Read the model definition and answer for the solid it produces. Units are mm, in the model's axes. A direction names the side the tool comes from. Give positions to 0.01 mm unless a question says otherwise; leave off trailing zeros. Write each loop counter-clockwise with the first axis right and the second up, starting at its lowest first coordinate (ties: lowest second). Pieces come first, ordered by that corner, then holes.
```python
from build123d import *

# Parameters (mm, degrees)
EXTRUDE_1_DEPTH               = 5
HOLE_WIZARD_M10_1_D           = 11
HOLE_WIZARD_M10_1_CBORE_D     = 12.05
HOLE_WIZARD_M10_1_CBORE_DEPTH = 4
HOLE_WIZARD_M10_2_D           = 11
HOLE_WIZARD_M10_2_CBORE_D     = 12.05
HOLE_WIZARD_M10_2_CBORE_DEPTH = 4
FILLET_1_R                    = 2


with BuildPart() as part:
    # 草图1 → 凸台-拉伸1 (new body)
    with BuildSketch(Plane(origin=(0, 0, 0), x_dir=(-1, 0, 0), z_dir=(0, 0, -1))):
        with BuildLine():
            Line((-3, 22.583801513), (-3, 7.416198487))
            ThreePointArc((-3, 7.416198487), (0, -8), (3, 7.416198487))
            Line((3, 7.416198487), (3, 22.583801513))
            ThreePointArc((3, 22.583801513), (0, 38), (-3, 22.583801513))
        make_face()
    extrude(amount=-EXTRUDE_1_DEPTH)

    # M10 六角头螺栓的柱形沉头孔1 (through all)
    with Locations(Plane(origin=(0, 0, 0), x_dir=(-1, 0, 0), z_dir=(0, 0, -1))):
        with Locations((0, 30)):
            CounterBoreHole(HOLE_WIZARD_M10_1_D / 2, HOLE_WIZARD_M10_1_CBORE_D / 2, HOLE_WIZARD_M10_1_CBORE_DEPTH)

    # M10 六角头螺栓的柱形沉头孔2 (through all)
    with Locations(Plane.XY.offset(5)):
        with Locations((0, 0)):
            CounterBoreHole(HOLE_WIZARD_M10_2_D / 2, HOLE_WIZARD_M10_2_CBORE_D / 2, HOLE_WIZARD_M10_2_CBORE_DEPTH)

    # 圆角1
    fillet_1_edges = [part.edges().sort_by_distance(p)[0] for p in [
        (-3, 22.583801513, 2.5),
        (-3, 7.416198487, 2.5),
        (3, 7.416198487, 2.5),
        (3, 22.583801513, 2.5),
    ]]
    fillet(fillet_1_edges, radius=FILLET_1_R)


solid = part.part
```
Item 1: Section D-D (y = 1.5) is taken. Write down the section's boundary in (x, z).
Result set:
outline: (-7.86, 0) - (-5.29, 0) - (-5.29, 1) - (-5.84, 1) - (-5.84, 5) - (-7.86, 5) - close; (5.29, 0) - (7.86, 0) - (7.86, 5) - (5.84, 5) - (5.84, 1) - (5.29, 1) - close
Item 2: Each of these flat-tipped pins is pushed along its axis until it touches: pin 1 Ø9.5 at (x, y) = (0, 0) entering from +Z; pin 2 Ø1 at (x, z) = (-3.5, 4.5) entering from -Y; pin 3 Ø1.5 at (y, z) = (23.5, 3) entering from -X. Where does it stop, or does it pass through?
Result set:
pin 1: passes through
pin 2: stops at y = -7.42
pin 3: stops at x = -5.56
Item 3: Section C-C (z = 4.6) is taken. Write down the section's boundary in (x, y) (3 decimals).
Result set:
outline: (-4, 6.928) arc R8 ccw (long way) to (4, 6.928) arc R2 cw to (3, 8.66) - (3, 21.34) arc R2 cw to (4, 23.072) arc R8 ccw (long way) to (-4, 23.072) arc R2 cw to (-3, 21.34) - (-3, 8.66) arc R2 cw to start; hole circle Ø12.05 at (0, 0); hole circle Ø11 at (0, 30)
Item 4: Section B-B (x = 0) is taken. Write down the section's boundary in (y, z) (3 decimals).
Result set:
outline: (-8, 0) - (-5.5, 0) - (-5.5, 1) - (-6.025, 1) - (-6.025, 5) - (-8, 5) - close; (5.5, 0) - (23.975, 0) - (23.975, 4) - (24.5, 4) - (24.5, 5) - (6.025, 5) - (6.025, 1) - (5.5, 1) - close; (35.5, 4) - (36.025, 4) - (36.025, 0) - (38, 0) - (38, 5) - (35.5, 5) - close
Item 5: Section A-A (y = 30) is taken. Write down the section's boundary in (x, z) (3 decimals), and give its area (3 significant figures).
Result set:
outline: (-8, 0) - (-6.025, 0) - (-6.025, 4) - (-5.5, 4) - (-5.5, 5) - (-8, 5) - close; (5.5, 4) - (6.025, 4) - (6.025, 0) - (8, 0) - (8, 5) - (5.5, 5) - close
area: 20.8 mm2
Item 6: Find the intervals of material crossed by line 1 along Y through (x, z) = (0, 4.1) (3 decimals); line 2 along Y through (x, z) = (0, 1.3) (3 decimals); line 3 along Y through (x, z) = (-6.75, 1.15), in increasing order.
Result set:
line 1: y = -8 to -6.025, 6.025 to 24.5, 35.5 to 38
line 2: y = -8 to -6.025, 6.025 to 23.975, 36.025 to 38
line 3: y = -4.29 to 4.29, 25.71 to 34.29
Item 7: Which of the six approach directions +Z, -Z, +X, -X, +Y, -Y give full straight-line access (tool end or side, diameter ignored) to faces 1 (the flat face through (3, -5, 1)), 2 (the cylindrical face through (-3.275, 22.352, 2.535)), 3 (the flat face through (3, 15, 2))?
Result set:
face 1: +Z
face 2: +Z, -Z, -X
face 3: +Z, -Z, +X
Item 8: Determine the mould class of faces 4 (the cylindrical face through (-0.716, 35.453, 4.507)), 5 (the flat face through (0, 15, 5)) for opening direction Y: pulls with the +Y half, pulls with the -Y half, needs draft (parallel to the pull), parting line crosses it, or undercut.
Result set:
face 4: undercut
face 5: needs draft
